Autodesk Inventor part; units mm, degrees
ref_plane "YZ Plane" through (0, 0, 0) normal (1, 0, 0) x (0, 1, 0)
ref_plane "XZ Plane" through (0, 0, 0) normal (0, 1, 0) x (-1, 0, 0)
ref_plane "XY Plane" through (0, 0, 0) normal (0, 0, 1) x (1, 0, 0)
sketch "Sketch1" plane through (0, 0, 0) normal (1, 0, 0) x (0, 1, 0)
  line L0 (21.7077, 51.1019) -> (7.4012, 36.7954)
  line L1 (7.4012, 36.7954) -> (7.4012, 0)
  line L2 (21.7077, 51.1019) -> (21.7077, 0)
  line L3 (7.4012, -36.7954) -> (7.4012, 0)
  line L4 (21.7077, -51.1019) -> (21.7077, 0)
  line L5 (21.7077, -51.1019) -> (7.4012, -36.7954)
  line L6 (21.7077, -51.1019) -> (21.7077, 51.1019)
  line L7 (17.1717, -14.2524) -> (13.4217, -14.2524)
  line L8 (13.4217, -14.2524) -> (11.5467, -17.5)
  line L9 (19.0467, -17.5) -> (17.1717, -14.2524)
  circle A0 centre (15.2967, -17.5) radius 3.75
  line L10 (17.1717, -20.7476) -> (19.0467, -17.5)
  line L11 (11.5467, -17.5) -> (13.4217, -20.7476)
  line L12 (13.4217, -20.7476) -> (17.1717, -20.7476)
  line L13 (17.1717, -31.7524) -> (13.4217, -31.7524)
  line L14 (19.0467, -35) -> (17.1717, -31.7524)
  line L15 (13.4217, -31.7524) -> (11.5467, -35)
  line L16 (13.4217, -38.2476) -> (17.1717, -38.2476)
  line L17 (17.1717, -38.2476) -> (19.0467, -35)
  line L18 (11.5467, -35) -> (13.4217, -38.2476)
  circle A1 centre (15.2967, -35) radius 3.75
  circle A2 centre (15.2967, 0) radius 3.75
  line L19 (13.4217, -3.2476) -> (17.1717, -3.2476)
  line L20 (17.1717, -3.2476) -> (19.0467, 0)
  line L21 (11.5467, 0) -> (13.4217, -3.2476)
  line L22 (13.4217, 3.2476) -> (11.5467, 0)
  line L23 (17.1717, 3.2476) -> (13.4217, 3.2476)
  line L24 (19.0467, 0) -> (17.1717, 3.2476)
  line L25 (13.4217, 14.2524) -> (17.1717, 14.2524)
  line L26 (11.5467, 17.5) -> (13.4217, 14.2524)
  line L27 (17.1717, 14.2524) -> (19.0467, 17.5)
  circle A3 centre (15.2967, 17.5) radius 3.75
  line L28 (19.0467, 17.5) -> (17.1717, 20.7476)
  line L29 (17.1717, 20.7476) -> (13.4217, 20.7476)
  line L30 (13.4217, 20.7476) -> (11.5467, 17.5)
  circle A4 centre (15.2967, 35) radius 3.75
  line L31 (13.4217, 31.7524) -> (17.1717, 31.7524)
  line L32 (11.5467, 35) -> (13.4217, 31.7524)
  line L33 (17.1717, 31.7524) -> (19.0467, 35)
  line L34 (19.0467, 35) -> (17.1717, 38.2476)
  line L35 (13.4217, 38.2476) -> (11.5467, 35)
  line L36 (17.1717, 38.2476) -> (13.4217, 38.2476)
  line L37 (21.7077, 47.5664) -> (7.4012, 33.2599)
  line L38 (9.9012, 39.2954) -> (9.9012, -39.2954)
  line L39 (7.4012, -33.2599) -> (21.7077, -47.5664)
  line L40 (15.2967, 35) -> (9.9012, 35)
  line L41 (9.9012, 26.25) -> (16.1703, 26.25)
  circle A5 centre (12.9012, 26.25) radius 2
  line L42 (9.9012, 23.25) -> (15.9012, 23.25)
  line L43 (15.9012, 23.25) -> (15.9012, 29.25)
  line L44 (15.9012, 29.25) -> (9.9012, 29.25)
  line L45 (9.9012, 29.25) -> (9.9012, 23.25)
  line L46 (9.9012, 23.25) -> (15.9012, 29.25) construction
  line L47 (15.9012, 23.25) -> (9.9012, 29.25) construction
  line L48 (9.9012, -26.25) -> (17.1717, -26.25)
  circle A6 centre (12.9012, -26.25) radius 2
  line L49 (15.9012, -29.25) -> (9.9012, -29.25)
  line L50 (9.9012, -29.25) -> (9.9012, -23.25)
  line L51 (9.9012, -23.25) -> (15.9012, -23.25)
  line L52 (15.9012, -23.25) -> (15.9012, -29.25)
  line L53 (15.9012, -29.25) -> (9.9012, -23.25) construction
  line L54 (9.9012, -29.25) -> (15.9012, -23.25) construction
  line L55 (15.9012, 53.3729) -> (15.9012, -51.1019)
  line L56 (9.9012, 26.25) -> (7.4012, 26.25)
  line L57 (14.9012, -60.8562) -> (14.9012, 66.1701)
  point P0 (9.9012, 35.7599)
  point P1 (9.9012, -35.7599)
  point P2 (14.9012, 40.7599)
  point P3 (14.9012, 44.2954)
  point P4 (14.9012, -44.2954)
  point P5 (14.9012, -40.7599)
  dimension "d33" = 2.5
  dimension "d34" = 2.5
  dimension "d35" = 2.5
  dimension "d36" = 8.75
  dimension "d37" = 4
  dimension "d38" = 3
  dimension "d39" = 6
  dimension "d40" = 8.75
  dimension "d41" = 4
  dimension "d42" = 3
  dimension "d43" = 6
  dimension "d48" = 8.5
  dimension "d49" = 7.5
extrude "Extrusion1" add sketch "Sketch1" along normal blind 3.5 contours L38 L37 L1 L0 | L0 L57 L37 L38 | L38 L56 L1 L37 | L56 L38 L39 L3 L1 | L44 L57 A5 L41 L38 | L41 A5 L57 L42 L38 | L44 L43 L41 L57 | L39 L38 L5 L3 | L41 L43 L42 L57 | L39 L57 L5 L38 | L51 L57 A6 L48 L38 | L38 L48 A6 L57 L49 | L51 L52 L48 L57 | L57 L48 L52 L49
sketch "Sketch2" plane through (3.5, 0, 0) normal (1, 0, 0) x (0, 0, -1)
  line L0 (-44.2954, 14.9012) -> (-36.7954, 7.4012)
  line L1 (-36.7954, 7.4012) -> (36.7954, 7.4012)
  line L2 (36.7954, 7.4012) -> (44.2954, 14.9012)
  line L3 (40.7599, 14.9012) -> (35.7599, 9.9012)
  line L4 (35.7599, 9.9012) -> (29.25, 9.9012)
  line L5 (29.25, 9.9012) -> (29.25, 15.9012)
  line L6 (29.25, 15.9012) -> (23.25, 15.9012)
  line L7 (23.25, 15.9012) -> (23.25, 9.9012)
  line L8 (23.25, 9.9012) -> (-23.25, 9.9012)
  line L9 (-23.25, 9.9012) -> (-23.25, 15.9012)
  line L10 (-23.25, 15.9012) -> (-29.25, 15.9012)
  line L11 (-29.25, 15.9012) -> (-29.25, 9.9012)
  line L12 (-29.25, 9.9012) -> (-35.7599, 9.9012)
  line L13 (-35.7599, 9.9012) -> (-40.7599, 14.9012)
  circle A0 centre (-26.25, 12.9012) radius 2
  circle A1 centre (26.25, 12.9012) radius 2
  line L14 (-29.25, 9.9012) -> (-23.25, 9.9012)
  line L15 (35.7599, 9.9012) -> (29.25, 9.9012)
  line L16 (23.25, 15.9012) -> (23.25, 9.9012)
  line L17 (29.25, 9.9012) -> (23.25, 9.9012)
  line L18 (-40.7599, 14.9012) -> (-44.2954, 14.9012)
  line L19 (44.2954, 14.9012) -> (40.7599, 14.9012)
  point P0 (0, 0)
extrude "Extrusion2" add sketch "Sketch2" along normal blind 29 contours L18 L13 L12 L14 L8 L17 L4 L3 L19 L2 L1 L0
mirror "Mirror1" about plane through (32.5, 11.1512, 0) normal (1, 0, 0)
sketch "Sketch4" plane through (0, 9.9012, 23.25) normal (0, 1, 0) x (1, 0, 0)
  line L0 (0, 59.0099) -> (0, 52.5)
  line L1 (0, 52.5) -> (3.5, 52.5)
  line L2 (3.5, 46.5) -> (3.5, 52.5)
  line L3 (0, 46.5) -> (3.5, 46.5)
  line L4 (0, 46.5) -> (0, 0)
  line L5 (0, 0) -> (3.5, 0)
  line L6 (3.5, -6) -> (3.5, 0)
  line L7 (0, -6) -> (3.5, -6)
  line L8 (0, -6) -> (0, -12.5099)
  line L9 (0, -12.5099) -> (65, -12.5099)
  line L10 (65, -6) -> (65, -12.5099)
  line L11 (65, -6) -> (61.5, -6)
  line L12 (61.5, -6) -> (61.5, 0)
  line L13 (65, 0) -> (61.5, 0)
  line L14 (65, 46.5) -> (65, 0)
  line L15 (65, 46.5) -> (61.5, 46.5)
  line L16 (61.5, 46.5) -> (61.5, 52.5)
  line L17 (65, 52.5) -> (61.5, 52.5)
  line L18 (65, 59.0099) -> (65, 52.5)
  line L19 (0, 59.0099) -> (65, 59.0099)
  line L20 (0, 52.5) -> (65, 52.5)
  line L21 (65, -13.5454) -> (65, 60.0454)
  line L22 (0, -6) -> (65, -6)
  line L23 (0, 52.5) -> (65, -6)
  line L24 (0, -6) -> (3.5, -6)
  line L25 (0, -6) -> (65, 52.5)
  line L26 (32.5, 52.5) -> (32.5, -6)
  line L27 (65, 46.5) -> (65, 0)
  line L28 (65, 23.25) -> (0, 23.25)
  line L29 (65, 23.25) -> (32.5, 52.5)
  line L30 (0, 23.25) -> (32.5, 52.5)
  line L31 (0, 23.25) -> (32.5, -6)
  line L32 (32.5, -6) -> (65, 23.25)
  circle A0 centre (16.25, 37.875) radius 7.5
  circle A1 centre (32.5, 23.25) radius 7.5
  circle A2 centre (48.75, 37.875) radius 7.5
  circle A3 centre (16.25, 8.625) radius 7.5
  circle A4 centre (48.75, 8.625) radius 7.5
  line L33 (16.25, 59.0099) -> (16.25, -12.5099)
  line L34 (0, -12.5099) -> (65, -12.5099)
  line L35 (48.75, -12.5099) -> (48.75, 59.0099)
  line L36 (0, 59.0099) -> (65, 59.0099)
  line L37 (32.5, 59.0099) -> (32.5, -12.5099)
  circle A5 centre (32.5, 52.5) radius 5
  circle A6 centre (32.5, -6) radius 5
  arc A7 (0, 15.75) -> (0, 30.75) centre (0, 23.25) ccw
  arc A8 (65, 30.75) -> (65, 15.75) centre (65, 23.25) ccw
  dimension "d62" = 15
  dimension "d63" = 15
  dimension "d64" = 15
  dimension "d65" = 15
  dimension "d66" = 15
  dimension "d69" = 10
  dimension "d70" = 10
  dimension "d71" = 15
  dimension "d72" = 15
extrude "Extrusion3" cut sketch "Sketch4" against normal blind 10 contours A0 L33 L23 | L23 L30 A0 | A5 L20 L37 | L37 L20 A5 | L20 L30 A5 | A0 L30 L33 | L30 A0 L23 | L33 A0 L30 | L23 A0 L33 | L29 A5 L26 | L20 A5 L29 | L26 A5 L30 | A7 L30 L4 | A7 L28 L30 | L35 L29 A2 | A2 L25 L35 | L31 A7 L4 | L28 A7 L31 | A1 L26 L23 | L23 L28 A1 | A2 L29 L25 | L29 L25 A2 | L35 A2 L25 | L29 A2 L35 | A1 L25 L26 | L28 A1 L23 | L26 A1 L25 | L23 A1 L26 | L25 A1 L28 | L25 A1 L28 | L33 L31 A3 | A3 L25 L33 | L14 L29 A8 | L31 L25 A3 | A3 L31 L25 | L33 A3 L25 | L31 A3 L33 | L32 A8 L28 | L28 A8 L29 | L14 A8 L32 | A4 L35 L23 | L23 L32 A4 | A6 L32 L26 | L26 L31 A6 | A4 L32 L35 | L32 A4 L23 | L35 A4 L32 | L23 A4 L35 | L32 A6 L22 | L37 A6 L22 | L22 A6 L31 | L22 A6 L37
properties part number "Bed"
Source: CAD feature listing. Evaluate the final solid. Frame: model axes, mm. A direction names the side the tool comes from. Round coordinates to 2 decimals unless told otherwise and drop trailing zeros. Write each loop counter-clockwise with the first axis right and the second up, starting at its lowest first coordinate (ties: lowest second). Pieces come first, ordered by that corner, then holes. Notation, with made-up numbers: M -35.5,64 L -17.5,64 A22 cw -17.5,72 Z; hole C 52.25,-18 d10. An arc over 180 degrees is marked long. Answer as a JSON object with one key per item and string values. Group by question number.
(1) Section query C-C on z = -17.5. Output: boundary loops of the cut face in (x, y).
(2) First-contact query: pin 1 (6 mm diameter, centred on x = 32.5, z = -29.25, fed in from -Y); pin 2 (1.8 mm diameter, centred on x = 2, y = 13.5, fed in from -Z); pin 3 (3 mm diameter, centred on x = 43.5, z = -42.5, fed in from +Y); pin 4 (17 mm diameter, centred on x = 48.75, z = 14.625, fed in from +Y). Flat tips, straight axial feed; report the tip coordinate or a pass-through.
(3) Section query A-A on z = 26.25. Output: boundary loops of the cut face in (x, y).
(4) Mould query, pull axis Z, two halves, no side actions, for faces 1 (the flat face through (32.045, 11.204, 40.598)), 2 (the flat face through (63, 13, -29.25)), 3 (the flat face through (65, 10, 26)). Classes: +Z half, -Z half, draft (parallel to the pull), parting line (faces both ways), or undercut.
(5) Section query B-B on x = 32.5. Output: boundary loops of the cut face in (y, z), then the cut area to 3 significant figures.
(6) Ray query, line 1 (Z direction, x = 16.25, y = 8.7) (3 decimals); line 2 (Z direction, x = 12, y = 9.75); line 3 (X direction, y = 8, z = -20). Return the intervals inside material, ascending. Write a range as [from, to].
(7) Reachability of faces 4 (the flat face through (61.5, 15, 27)), 5 (the cylindrical face through (1.726, 11.314, -25.033)), 6 (the flat face through (32.045, 12.436, -38.295)) from +Z, -Z, +X, -X, +Y, -Y: full face, straight path, thin tool, end or side. Return the list, or none.
(8) Section query D-D on x = 26. Output: boundary loops of the cut face in (y, z).
Computed values:
{
 "1": {"outline": "M 0,7.4 L 9.32,7.4 L 9.32,9.9 L 0,9.9 Z; M 23.18,7.4 L 41.82,7.4 L 41.82,9.9 L 23.18,9.9 Z; M 55.68,7.4 L 65,7.4 L 65,9.9 L 55.68,9.9 Z"},
 "2": {"pin 1": "through", "pin 2": "z = -43.79", "pin 3": "y = 14.9", "pin 4": "y = 9.9"},
 "3": {"outline": "M 0,7.4 L 28.5,7.4 L 28.5,9.9 L 3.5,9.9 L 3.5,10.9 L 0,10.9 Z; M 0,14.9 L 3.5,14.9 L 3.5,15.9 L 0,15.9 Z; M 36.5,7.4 L 65,7.4 L 65,10.9 L 61.5,10.9 L 61.5,9.9 L 36.5,9.9 Z; M 61.5,14.9 L 65,14.9 L 65,15.9 L 61.5,15.9 Z"},
 "4": {"face 1": "+Z half", "face 2": "undercut", "face 3": "draft"},
 "5": {"outline": "M 7.4,-36.8 L 14.9,-44.3 L 14.9,-40.76 L 9.9,-35.76 L 9.9,-34.25 L 7.4,-34.25 Z; M 7.4,-24.25 L 9.9,-24.25 L 9.9,-7.5 L 7.4,-7.5 Z; M 7.4,7.5 L 9.9,7.5 L 9.9,24.25 L 7.4,24.25 Z; M 7.4,34.25 L 9.9,34.25 L 9.9,35.76 L 14.9,40.76 L 14.9,44.3 L 7.4,36.8 Z", "area": "138 mm^2"},
 "6": {"line 1": "[-38.094, -22.125], [-7.125, 7.125], [22.125, 38.094]", "line 2": "[-39.14, -20.8], [-8.45, 8.45], [20.8, 39.14]", "line 3": "[0, 11.02], [21.48, 43.52], [53.98, 65]"},
 "7": {"face 4": "+Y", "face 5": "+X, -X", "face 6": "+X, -X, +Y"},
 "8": {"outline": "M 7.4,-36.8 L 14.9,-44.3 L 14.9,-40.76 L 9.9,-35.76 L 9.9,-3.74 L 7.4,-3.74 Z; M 7.4,3.74 L 9.9,3.74 L 9.9,35.76 L 14.9,40.76 L 14.9,44.3 L 7.4,36.8 Z"}
}
